```python
from build123d import *

# Parameters (mm, degrees)
SKETCH_1_W      = 44
SKETCH_1_H      = 37
SKETCH_1_R      = 1.5
SKETCH_1_W_2    = 12
SKETCH_1_H_2    = 5
EXTRUDE_1_DEPTH = 5.86


with BuildPart() as part:
    # 草图1 → 凸台-拉伸1 (new body)
    # profile 1 of 2: a face of its own
    with BuildSketch(Plane(origin=(0, 0, 0), x_dir=(1, 0, 0), z_dir=(0, 1, 0))):
        Rectangle(SKETCH_1_W, SKETCH_1_H)
        with Locations(Location((-15.25, -15.25, 0), (0, 0, 90))):
            Circle(SKETCH_1_R, mode=Mode.SUBTRACT)
        with Locations(Location((15.25, -15.25, 0), (0, 0, 90))):
            Circle(SKETCH_1_R, mode=Mode.SUBTRACT)
        with Locations(Location((15.25, 15.25, 0), (0, 0, 90))):
            Circle(SKETCH_1_R, mode=Mode.SUBTRACT)
        with Locations(Location((-15.25, 15.25, 0), (0, 0, 90))):
            Circle(SKETCH_1_R, mode=Mode.SUBTRACT)
    # profile 2 of 2: a face of its own
    with BuildSketch(Plane(origin=(0, 0, 0), x_dir=(1, 0, 0), z_dir=(0, 1, 0))):
        with Locations((0, -21)):
            Rectangle(SKETCH_1_W_2, SKETCH_1_H_2)
    extrude(amount=EXTRUDE_1_DEPTH)


solid = part.part
```
Model file for the job. Use its own axes, mm. A direction names the side the tool comes from. Give positions to 0.01 mm unless a question says otherwise; leave off trailing zeros. Write each loop counter-clockwise with the first axis right and the second up, starting at its lowest first coordinate (ties: lowest second). Pieces come first, ordered by that corner, then holes. Notation, with made-up numbers: M 73,30 L 106,30 A17 ccw 106,63 Z; hole C -11,17 d11. An arc over 180 degrees is marked long. Use a Markdown table: item, result.
1) Drill centre lines: line 1 (X direction, y = 4.5, z = -15.25); line 2 (Z direction, x = 15.25, y = 1.5); line 3 (Z direction, x = -14, y = 5.25). Where is each one in solid material? Low to high. Write a range as from..to.
Responses:
| item | result |
|---|---|
| line 1 | x = -22..-16.75, -13.75..13.75, 16.75..22 |
| line 2 | z = -18.5..-16.75, -13.75..13.75, 16.75..18.5 |
| line 3 | z = -18.5..-16.08, -14.42..14.42, 16.08..18.5 |
2) Cut at C-C (x = -15.25). List the corners of the cut face in (y, z).
Responses:
| item | result |
|---|---|
| outline | M 0,-18.5 L 5.86,-18.5 L 5.86,-16.75 L 0,-16.75 Z; M 0,-13.75 L 5.86,-13.75 L 5.86,13.75 L 0,13.75 Z; M 0,16.75 L 5.86,16.75 L 5.86,18.5 L 0,18.5 Z |
3) Pin check, flat tips, straight feed: pin 1 (2.5 mm diameter, centred on y = 3, z = 22, fed in from +X); pin 2 (1.8 mm diameter, centred on x = 10, y = 2.5, fed in from +Z); pin 3 (1.8 mm diameter, centred on x = 15.25, z = 15.25, fed in from -Y). Stop position of each tip, or through.
Responses:
| item | result |
|---|---|
| pin 1 | stops at x = 6 |
| pin 2 | stops at z = 18.5 |
| pin 3 | passes through |
4) Tool access for faces 4 (the cylindrical face through (-15.32, 2.89, 16.75)), 5 (the flat face through (-14, 3, 18.5)): list every direction of +Z, -Z, +X, -X, +Y, -Y with a clear straight run to the whole face (end or side of a thin tool).
Responses:
| item | result |
|---|---|
| face 4 | +Y, -Y |
| face 5 | +Z, -X, +Y, -Y |
5) Pull direction X, two halves, no side cores. Call faces 1 (the flat face through (6, 3, 21)), 2 (the cylindrical face through (-15.32, 2.89, -13.75)), 3 (the flat face through (14, 3, 18.5)): +X half, -X half, draft (parallel to the pull), parting line (faces both ways), or undercut.
Responses:
| item | result |
|---|---|
| face 1 | +X half |
| face 2 | undercut |
| face 3 | draft |
6) Cut at A-A (z = -15.25). List the corners of the cut face in (x, y).
Responses:
| item | result |
|---|---|
| outline | M -22,0 L -16.75,0 L -16.75,5.86 L -22,5.86 Z; M -13.75,0 L 13.75,0 L 13.75,5.86 L -13.75,5.86 Z; M 16.75,0 L 22,0 L 22,5.86 L 16.75,5.86 Z |
7) Cut at B-B (y = 3.65). List the corners of the cut face in (x, z).
Responses:
| item | result |
|---|---|
| outline | M -22,-18.5 L 22,-18.5 L 22,18.5 L 6,18.5 L 6,23.5 L -6,23.5 L -6,18.5 L -22,18.5 Z; hole C -15.25,-15.25 d3; hole C -15.25,15.25 d3; hole C 15.25,-15.25 d3; hole C 15.25,15.25 d3 |
